Model file for the job. Use its own axes, mm. Round coordinates to 2 decimals unless told otherwise and drop trailing zeros. Order: outer loops, then holes, each group sorted by start corner. A loop starts at its lowest first (then second) coordinate and runs counter-clockwise, first axis right, second up. Notation, with made-up numbers: (81.25, 32) -> (135.25, 32) arc R20 ccw to (135.25, 48) -> close; hole circle Ø3 at (57, 31.25). An arc over 180 degrees is marked (long way). Use CSV: the item, a comma, the result in double quotes.
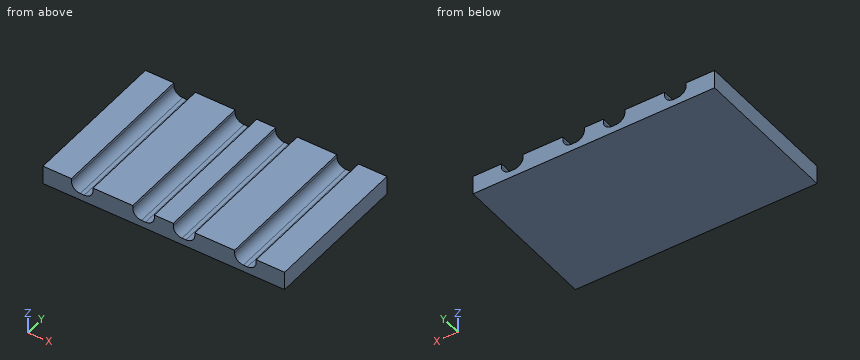
```python
from build123d import *

# Parameters (mm, degrees)
F1_DEPTH = 50.8


with BuildPart() as f1:
    # F0 (on Front) → F1 (new body)
    with BuildSketch(Plane.XZ):
        with BuildLine():
            Line((-31.4099, 74.034357), (-41.0718, 74.034357))
            Line((-41.0718, 74.034357), (-41.0718, 67.684357))
            Line((-41.0718, 67.684357), (41.0718, 67.684357))
            Line((41.0718, 67.684357), (41.0718, 74.034357))
            Line((41.0718, 74.034357), (31.4099, 74.034357))
            Line((31.4099, 74.034357), (31.4099, 73.034357))
            ThreePointArc((31.4099, 73.034357), (30.53122, 70.913037), (28.4099, 70.034357))
            Line((28.4099, 70.034357), (27.0637, 70.034357))
            ThreePointArc((27.0637, 70.034357), (24.94238, 70.913037), (24.0637, 73.034357))
            Line((24.0637, 73.034357), (24.0637, 74.034357))
            Line((24.0637, 74.034357), (10.5565, 74.034357))
            Line((10.5565, 74.034357), (10.5565, 73.924565))
            Line((10.5565, 73.924565), (10.5565, 73.034357))
            ThreePointArc((10.5565, 73.034357), (9.67782, 70.913037), (7.5565, 70.034357))
            Line((7.5565, 70.034357), (6.2103, 70.034357))
            ThreePointArc((6.2103, 70.034357), (4.08898, 70.913037), (3.2103, 73.034357))
            Line((3.2103, 73.034357), (3.2103, 74.034357))
            Line((3.2103, 74.034357), (-3.2103, 74.034357))
            Line((-3.2103, 74.034357), (-3.2103, 73.034357))
            ThreePointArc((-3.2103, 73.034357), (-4.08898, 70.913037), (-6.2103, 70.034357))
            Line((-6.2103, 70.034357), (-7.5565, 70.034357))
            ThreePointArc((-7.5565, 70.034357), (-9.67782, 70.913037), (-10.5565, 73.034357))
            Line((-10.5565, 73.034357), (-10.5565, 74.034357))
            Line((-10.5565, 74.034357), (-24.0637, 74.034357))
            Line((-24.0637, 74.034357), (-24.0637, 73.924565))
            Line((-24.0637, 73.924565), (-24.0637, 73.034357))
            ThreePointArc((-24.0637, 73.034357), (-24.94238, 70.913037), (-27.0637, 70.034357))
            Line((-27.0637, 70.034357), (-28.4099, 70.034357))
            ThreePointArc((-28.4099, 70.034357), (-30.53122, 70.913037), (-31.4099, 73.034357))
            Line((-31.4099, 73.034357), (-31.4099, 74.034357))
        make_face()
    extrude(amount=F1_DEPTH)


solid = f1.part
```
Q1. Cut at B-B (y = -23.5). Give the cut face in (x, z).
From the geometry:
outline,"(-41.07, 67.68) -> (41.07, 67.68) -> (41.07, 74.03) -> (31.41, 74.03) -> (31.41, 73.03) arc R3 cw to (28.41, 70.03) -> (27.06, 70.03) arc R3 cw to (24.06, 73.03) -> (24.06, 74.03) -> (10.56, 74.03) -> (10.56, 73.03) arc R3 cw to (7.56, 70.03) -> (6.21, 70.03) arc R3 cw to (3.21, 73.03) -> (3.21, 74.03) -> (-3.21, 74.03) -> (-3.21, 73.03) arc R3 cw to (-6.21, 70.03) -> (-7.56, 70.03) arc R3 cw to (-10.56, 73.03) -> (-10.56, 74.03) -> (-24.06, 74.03) -> (-24.06, 73.03) arc R3 cw to (-27.06, 70.03) -> (-28.41, 70.03) arc R3 cw to (-31.41, 73.03) -> (-31.41, 74.03) -> (-41.07, 74.03) -> close"
Q2. Probe line 1 along X through (y, z) = (-43, 72.75); line 2 along X through (y, z) = (-24, 73.75); line 3 along Z through (x, y) = (28.5, -20). List the from-to ranges inside material, lowest first.
From the geometry:
line 1,"x = -41.07 to -31.4, -24.08 to -10.54, -3.22 to 3.22, 10.54 to 24.08, 31.4 to 41.07"
line 2,"x = -41.07 to -31.41, -24.06 to -10.56, -3.21 to 3.21, 10.56 to 24.06, 31.41 to 41.07"
line 3,"z = 67.68 to 70.04"
Q3. Cut at C-C (x = 9). Give the cut face in (y, z), plus the area to 3 significant figures.
From the geometry:
outline,"(-50.8, 67.68) -> (0, 67.68) -> (0, 70.4) -> (-50.8, 70.4) -> close"
area,"138 mm²"
Q4. Cut at A-A (z = 72). Give the cut face in (x, y), plus the area to 3 significant figures.
From the geometry:
outline,"(-41.07, -50.8) -> (-31.23, -50.8) -> (-31.23, 0) -> (-41.07, 0) -> close; (-24.25, -50.8) -> (-10.37, -50.8) -> (-10.37, 0) -> (-24.25, 0) -> close; (-3.39, -50.8) -> (3.39, -50.8) -> (3.39, 0) -> (-3.39, 0) -> close; (10.37, -50.8) -> (24.25, -50.8) -> (24.25, 0) -> (10.37, 0) -> close; (31.23, -50.8) -> (41.07, -50.8) -> (41.07, 0) -> (31.23, 0) -> close"
area,"2,750 mm²"
Q5. Cut at D-D (x = 25). Give the cut face in (y, z), plus the area to 3 significant figures.
From the geometry:
outline,"(-50.8, 67.68) -> (0, 67.68) -> (0, 70.86) -> (-50.8, 70.86) -> close"
area,"161 mm²"
Q6. Pin check, flat tip, straight feed: pin 1 (1.1 mm diameter, centred on x = 27.5, y = -35.5, fed in from +Z). Stop position of the tip, or through.
From the geometry:
pin 1,"stops at z = 70.04"
